Autodesk Inventor part; units mm, degrees
ref_plane "YZ Plane" through (0, 0, 0) normal (1, 0, 0) x (0, 1, 0)
ref_plane "XZ Plane" through (0, 0, 0) normal (0, 1, 0) x (-1, 0, 0)
ref_plane "XY Plane" through (0, 0, 0) normal (0, 0, 1) x (1, 0, 0)
sketch "Sketch1" plane through (0, 0, 0) normal (0, 0, 1) x (1, 0, 0)
  line L0 (0, 0) -> (4, 0) construction
  line L1 (8, 0) -> (8, 7.1)
  line L2 (8, 7.1) -> (6.11, 7.1)
  line L3 (6.11, 7.1) -> (6.11, 14.1)
  line L4 (6.11, 14.1) -> (5.11, 14.1)
  line L5 (5.11, 14.1) -> (5.11, 15.1)
  line L6 (5.11, 15.1) -> (4, 15.1)
  line L7 (0, 15.1) -> (0, 0) construction
  line L8 (4, 15.1) -> (4, 0)
  line L9 (4, 15.1) -> (0, 15.1) construction
  line L10 (4, 0) -> (8, 0)
  dimension "d0" = 7
  dimension "d1" = 7.1
  dimension "d2" = 8
  dimension "d3" = 6.11
  dimension "d5" = 1
  dimension "d6" = 1
  dimension "d15" = 4
revolve "Revolution1" add sketch "Sketch1" angle 360 about axis through (0, 15.1, 0) along (0, -1, 0)
sketch "Sketch2" plane through (0, 14.1, 0) normal (0, 1, 0) x (1, 0, 0)
  circle A0 centre (0, 0) radius 5.11 construction
  line L0 (0, 0) -> (-6, 0) construction
  circle A1 centre (-6, 0) radius 0.6
  point P0 (0, 0)
  dimension "d8" = 1.2
  dimension "d9" = 6
extrude "Extrusion1" cut sketch "Sketch2" against normal up to surface (7 mm away)
pattern_circular "Circular Pattern1" count 20 over 360 about axis through (0, 14.6, 0) along (0, -1, 0) of "Extrusion1"
sketch "Sketch3" plane through (0, 0, 0) normal (1, 0, 0) x (0, 1, 0)
  line L0 (7.1, 8) -> (7.1, -8) construction
  line L1 (0, 8) -> (0, -8) construction
  line L2 (0, 0) -> (7.1, 0) construction
  circle A0 centre (3.55, 0) radius 1.25
  dimension "d16" = 2.5
extrude "Extrusion2" cut sketch "Sketch3" against normal blind 10
pattern_circular "Circular Pattern2" count 2 over 90 about axis through (0, 7.55, 0) along (0, -1, 0) of "Extrusion2"
properties part number "GT2Pulley_20T_8mm"
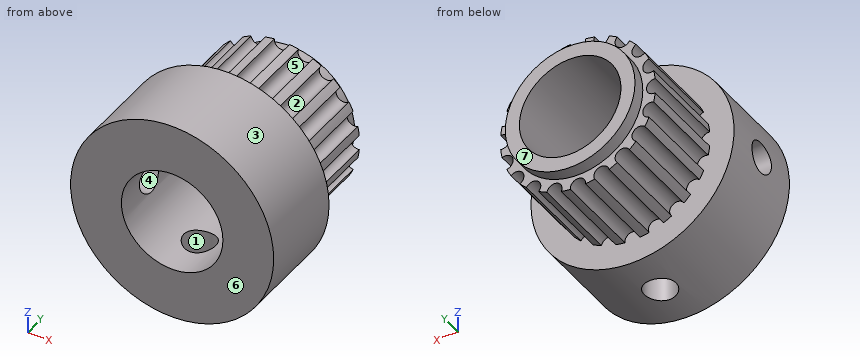
Work out the finished part from the listing and answer in its coordinate system (mm). Face numbers are marked on the shaded views. A direction names the side the tool comes from. Round coordinates to 2 decimals unless told otherwise and drop trailing zeros. Write each loop counter-clockwise with the first axis right and the second up, starting at its lowest first coordinate (ties: lowest second). Pieces come first, ordered by that corner, then holes. Notation, with made-up numbers: (-27, -17.75) - (-10, -17.75) arc R22 cw to (-10, 17.25) - close; hole circle Ø1 at (-0.5, -15). An arc over 180 degrees is marked (long way). Answer in a Markdown table with one row per item. Add a question column.
1. Given pin 1 (6.5 mm diameter, centred on x = 0, z = 0, fed in from -Y); pin 2 (1.6 mm diameter, centred on x = 3.53, z = -4.85, fed in from +Y); pin 3 (1.1 mm diameter, centred on x = 5.71, z = 1.85, fed in from +Y); pin 4 (3 mm diameter, centred on x = -4, y = 6, fed in from +Z), each flat-ended and moving along its own axis, determine where each tip first touches the part or whether it passes through.
2. Find the intervals of material crossed by line 1 along Y through (x, z) = (-2.5, 6.75); line 2 along Z through (x, y) = (1.25, 3); line 3 along Z through (x, y) = (-3.25, 3), in increasing order. Write a range as from..to.
3. A cutting plane is placed at B-B, the plane x = 0. Determine the outline of the cut face in (y, z).
4. The mould has two halves that part along Y. Classify the marked faces 4, 5, 6 and 7: +Y half, -Y half, draft (parallel to the pull), parting line (faces both ways), or undercut.
5. For the marked faces 1, 2 and 3, determine the directions among +Z, -Z, +X, -X, +Y, -Y from which every point of the face is accessible in a straight line to the end or side of a thin tool.
6. A cutting plane is placed at D-D, the plane x = 3.75. Determine the outline of the cut face in (y, z).
7. A cutting plane is placed at A-A, the plane z = 0. Determine the outline of the cut face in (x, y), and give its area (3 significant figures).
8. A cutting plane is placed at C-C, the plane y = 3.55. Determine the outline of the cut face in (x, z).
Worked out:
| question | item | result |
|---|---|---|
| 1 | pin 1 | through |
| 1 | pin 2 | y = 14.1 |
| 1 | pin 3 | y = 7.1 |
| 1 | pin 4 | z = 7.6 |
| 2 | line 1 | 0..7.1 |
| 2 | line 2 | -7.9..-3.8, 3.8..7.9 |
| 2 | line 3 | -7.31..-2.33, 2.33..7.31 |
| 3 | outline | (0, -8) - (2.3, -8) - (2.3, -4) - (0, -4) - close; (0, 4) - (15.1, 4) - (15.1, 5.11) - (14.1, 5.11) - (14.1, 5.4) - (7.1, 5.4) - (7.1, 8) - (0, 8) - close; (4.8, -8) - (7.1, -8) - (7.1, -5.4) - (14.1, -5.4) - (14.1, -5.11) - (15.1, -5.11) - (15.1, -4) - (4.8, -4) - close |
| 4 | face 4 | undercut |
| 4 | face 5 | draft |
| 4 | face 6 | -Y half |
| 4 | face 7 | +Y half |
| 5 | face 1 | -Z |
| 5 | face 2 | +Y |
| 5 | face 3 | +Y, -Y |
| 6 | outline | (0, -7.07) - (7.1, -7.07) - (7.1, -4.3) - (14.1, -4.3) - (14.1, -3.47) - (15.1, -3.47) - (15.1, -1.39) - (0, -1.39) - close; (0, 1.39) - (15.1, 1.39) - (15.1, 3.47) - (14.1, 3.47) - (14.1, 4.3) - (7.1, 4.3) - (7.1, 7.07) - (0, 7.07) - close |
| 7 | outline | (-8, 0) - (-4, 0) - (-4, 2.3) - (-8, 2.3) - close; (-8, 4.8) - (-4, 4.8) - (-4, 15.1) - (-5.11, 15.1) - (-5.11, 14.1) - (-5.4, 14.1) - (-5.4, 7.1) - (-8, 7.1) - close; (4, 0) - (8, 0) - (8, 7.1) - (5.4, 7.1) - (5.4, 14.1) - (5.11, 14.1) - (5.11, 15.1) - (4, 15.1) - close |
| 7 | area | 68.6 mm^2 |
| 8 | outline | (-7.9, -1.25) arc R8 ccw to (-1.25, -7.9) - (-1.25, -3.8) arc R4 cw to (-3.8, -1.25) - close; (-7.9, 1.25) - (-3.8, 1.25) arc R4 cw (long way) to (1.25, -3.8) - (1.25, -7.9) arc R8 ccw (long way) to start |
